Here's how the part is built. I have some questions about the finished solid (model axes, mm). Face numbers are marked on the shaded views. A direction names the side the tool comes from. Give positions to 0.01 mm unless a question says otherwise; leave off trailing zeros. Order: outer loops, then holes, each group sorted by start corner. A loop starts at its lowest first (then second) coordinate and runs counter-clockwise, first axis right, second up.
from build123d import *

# Parameters (mm, degrees)
SKETCH_1_R      = 1.65
EXTRUDE_1_DEPTH = 3
EXTRUDE_2_DEPTH = 2.9
CHAMFER_1_SIZE  = 2.9
FILLET_1_R      = 1


with BuildPart() as part:
    # 草图1 → 凸台-拉伸1 (new body)
    with BuildSketch(Plane.XY):
        Polygon((-76.15, 37.05), (-23.614971157, 37.05), (31.485028843, -18.05), (76.15, -18.05), (76.15, -37.05), (23.614971157, -37.05), (-31.485028843, 18.05), (-76.15, 18.05), align=None)
        with Locations((-66.15, 27.55)):
            Circle(SKETCH_1_R, mode=Mode.SUBTRACT)
        with Locations((66.15, -27.55)):
            Circle(SKETCH_1_R, mode=Mode.SUBTRACT)
    extrude(amount=EXTRUDE_1_DEPTH)

    # 草图2 → 凸台-拉伸2 (add)
    with BuildSketch(Plane.XY.offset(3)):
        Polygon((-57.15, 33.95), (-57.15, 21.15), (-30.200966799, 21.15), (24.899033201, -33.95), (57.15, -33.95), (57.15, -21.15), (30.200966799, -21.15), (-24.899033201, 33.95), align=None)
    extrude(amount=EXTRUDE_2_DEPTH)

    # 倒角1
    chamfer_1_edges = [part.edges().sort_by_distance(p)[0] for p in [
        (57.15, -27.55, 5.9),
        (-57.15, 27.55, 5.9),
    ]]
    chamfer(chamfer_1_edges, length=CHAMFER_1_SIZE - 0.0001)  # a hair under: the kernel refuses the full size

    # 圆角1
    fillet_1_edges = [part.edges().sort_by_distance(p)[0] for p in [
        (-23.614971157, 37.05, 1.5),
        (31.485028843, -18.05, 1.5),
        (23.614971157, -37.05, 1.5),
        (-31.485028843, 18.05, 1.5),
        (-24.899033201, 33.95, 4.45),
        (-30.200966799, 21.15, 4.45),
        (24.899033201, -33.95, 4.45),
        (30.200966799, -21.15, 4.45),
    ]]
    fillet(fillet_1_edges, radius=FILLET_1_R)


solid = part.part
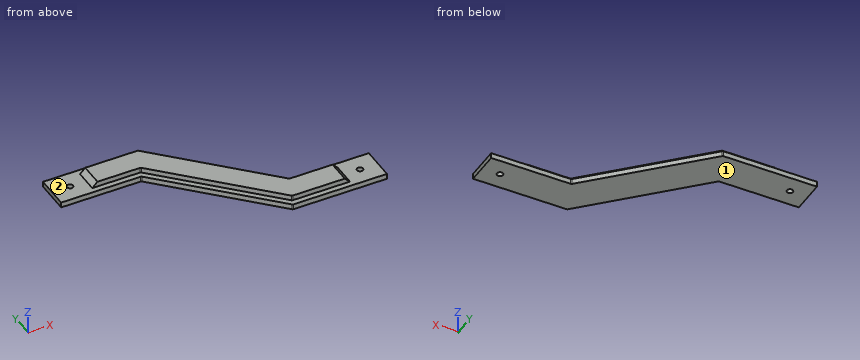
Q1. If we section it at D-D on y = -6: List the corners of the cut face in (x, z) for me.
Filled sheet:
outline: (-7.44, 0) - (19.44, 0) - (19.44, 3) - (15.05, 3) - (15.05, 5.9) - (-3.05, 5.9) - (-3.05, 3) - (-7.44, 3) - close
Q2. For the marked faces 1 and 2, which set-ups out of +Z, -Z, +X, -X, +Y, -Y let a thin tool reach every point of the face, with its end or its side?
Filled sheet:
face 1: -Z, +X, -X, +Y, -Y
face 2: +Z
Q3. I'm going to push flat-ended pins straight in: P1, Ø2.5, axis at x = 38, z = 5, coming from the -Y side; P2, Ø2.5, axis at x = 46.5, z = 4.5, coming from the +Y side; P3, Ø0.9, axis at x = -34, z = 4.5, coming from the +Y side; P4, Ø4.5, axis at x = -66.15, y = 27.55, coming from the -Z side. Where does each tip first touch, or does it pass through?
Filled sheet:
P1: stops at y = -33.95
P2: stops at y = -21.15
P3: stops at y = 33.95
P4: stops at z = 0
Q4. I need wall thicknesses on L1, parallel to Y at x = 66.15, z = 2.25; L2, parallel to Y at x = -66.15, z = 1.9; L3, parallel to Z at x = 19, y = -32. Which ranges of each line are inside material? Lowest first, please.
Filled sheet:
L1: y = -37.05 to -29.2, -25.9 to -18.05
L2: y = 18.05 to 25.9, 29.2 to 37.05
L3: z = 0 to 3
Q5. If we section it at C-C on x = 43: List the corners of the cut face in (y, z) for me, plus the area to 3 significant figures.
Filled sheet:
outline: (-37.05, 0) - (-18.05, 0) - (-18.05, 3) - (-21.15, 3) - (-21.15, 5.9) - (-33.95, 5.9) - (-33.95, 3) - (-37.05, 3) - close
area: 94.1 mm2
Q6. If we section it at A-A on x = -66.15: List the corners of the cut face in (y, z) for me, plus the area to 3 significant figures.
Filled sheet:
outline: (18.05, 0) - (25.9, 0) - (25.9, 3) - (18.05, 3) - close; (29.2, 0) - (37.05, 0) - (37.05, 3) - (29.2, 3) - close
area: 47.1 mm2
